Read the model definition and answer for the solid it produces. Units are mm, in the model's axes. Face numbers are marked on the shaded views. Coordinates: 2 decimals unless noted, no trailing zeros. Write each loop counter-clockwise with the first axis right and the second up, starting at its lowest first coordinate (ties: lowest second). Pieces come first, ordered by that corner, then holes.
(1) Section D-D on y = 5.5 is taken. Write down the section's boundary in (x, z), then the cut area to 3 significant figures.
(2) Section C-C on z = -12.25 is taken. Write down the section's boundary in (x, y), then the cut area to 3 significant figures.
(3) The mould has two halves that part along Z. Classify the marked faces 1, 2, 3 and 4: +Z half, -Z half, draft (parallel to the pull), parting line (faces both ways), or undercut.
(4) Section A-A on z = -21 is taken. Write down the section's boundary in (x, y).
(5) Find the intervals of material crossed by probe 1 along Z at (x, y) = (19.5, -16); probe 2 along Z at (x, y) = (-4.5, -15.5); probe 3 along X at (y, z) = (-28, -14), in increasing order.
(6) Given pin 1 (1 mm diameter, centred on y = 26.5, z = -11.5, fed in from -X); pin 2 (4.5 mm diameter, centred on y = -22, z = -20.5, fed in from -X); pin 3 (3 mm diameter, centred on x = -21.5, z = -19, fed in from +Y), each flat-ended and moving along its own axis, determine where each tip first touches the part or whether it passes through.
(7) Section B-B on x = 10.5 is taken. Write down the section's boundary in (y, z).
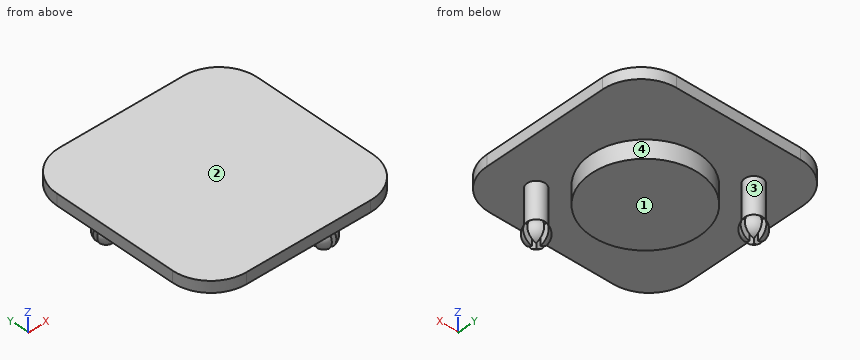
from build123d import *

# Parameters (mm, degrees)
BOX002_W     = 2
BOX002_H     = 12
BOX002_DEPTH = 10
BOX001_W     = 12
BOX001_H     = 2
BOX001_DEPTH = 10
BOX003_W     = 2
BOX003_H     = 12
BOX003_DEPTH = 10
BOX_W        = 12
BOX_H        = 2
BOX_DEPTH    = 10
PAD_DEPTH    = 5
SKETCH001_R  = 24
PAD001_DEPTH = 8
SKETCH002_R  = 4
PAD002_DEPTH = 16


with BuildPart() as cubo002:
    # Box002 → Box002 (new body)
    with BuildSketch(Plane(origin=(-26, 19, -25), x_dir=(1, 0, 0), z_dir=(0, 0, 1))):
        with Locations((1, 6)):
            Rectangle(BOX002_W, BOX002_H)
    extrude(amount=BOX002_DEPTH)


with BuildPart() as fusion:
    # Box001 → Box001 (new body)
    with BuildSketch(Plane(origin=(-31, 24, -25), x_dir=(1, 0, 0), z_dir=(0, 0, 1))):
        with Locations((6, 1)):
            Rectangle(BOX001_W, BOX001_H)
    extrude(amount=BOX001_DEPTH)

    # Fusion: union Cubo002
    add(cubo002.part)


with BuildPart() as cut001:
    # Sphere001 → Sphere001 (revolve)
    with BuildSketch(Plane(origin=(-25, 25, -19), x_dir=(1, 0, 0), z_dir=(0, -1, 0))):
        with BuildLine():
            ThreePointArc((0, -5), (5, 0), (0, 5))
            Line((0, 5), (0, -5))
        make_face()
    revolve(axis=Axis((-25, 25, -19), (0, 0, 1)))

    # Cut001: cut Fusion
    add(fusion.part, mode=Mode.SUBTRACT)


with BuildPart() as cubo003:
    # Box003 → Box003 (new body)
    with BuildSketch(Plane(origin=(24, -31, -25), x_dir=(1, 0, 0), z_dir=(0, 0, 1))):
        with Locations((1, 6)):
            Rectangle(BOX003_W, BOX003_H)
    extrude(amount=BOX003_DEPTH)


with BuildPart() as fusion001:
    # Box → Box (new body)
    with BuildSketch(Plane(origin=(19, -26, -25), x_dir=(1, 0, 0), z_dir=(0, 0, 1))):
        with Locations((6, 1)):
            Rectangle(BOX_W, BOX_H)
    extrude(amount=BOX_DEPTH)

    # Fusion001: union Cubo003
    add(cubo003.part)


with BuildPart() as cut:
    # Sphere → Sphere (revolve)
    with BuildSketch(Plane(origin=(25, -25, -19), x_dir=(1, 0, 0), z_dir=(0, -1, 0))):
        with BuildLine():
            ThreePointArc((0, -5), (5, 0), (0, 5))
            Line((0, 5), (0, -5))
        make_face()
    revolve(axis=Axis((25, -25, -19), (0, 0, 1)))

    # Cut: cut Fusion001
    add(fusion001.part, mode=Mode.SUBTRACT)


with BuildPart() as fusion002:
    # Sketch → Pad (new body)
    with BuildSketch(Plane.XY):
        with BuildLine():
            Line((-27.5, 44.5), (27.5, 44.5))
            ThreePointArc((44.5, 27.5), (39.520815, 39.520815), (27.5, 44.5))
            Line((44.5, 27.5), (44.5, -27.5))
            ThreePointArc((27.5, -44.5), (39.520815, -39.520815), (44.5, -27.5))
            Line((27.5, -44.5), (-27.5, -44.5))
            ThreePointArc((-44.5, -27.5), (-39.520815, -39.520815), (-27.5, -44.5))
            Line((-44.5, -27.5), (-44.5, 27.5))
            ThreePointArc((-27.5, 44.5), (-39.520815, 39.520815), (-44.5, 27.5))
        make_face()
    extrude(amount=PAD_DEPTH)

    # Sketch001 (on Face9 of Pad) → Pad001 (join)
    with BuildSketch(Plane(origin=(0, 0, 0), x_dir=(1, 0, 0), z_dir=(0, 0, -1))):
        with Locations((0.149781, -0.32649)):
            Circle(SKETCH001_R)
    extrude(amount=PAD001_DEPTH)

    # Sketch002 (on Face4 of Pad001) → Pad002 (join)
    with BuildSketch(Plane(origin=(0, 0, 0), x_dir=(1, 0, 0), z_dir=(0, 0, -1))):
        with Locations((25, 25)):
            Circle(SKETCH002_R)
        with Locations((-25, -25)):
            Circle(SKETCH002_R)
    extrude(amount=PAD002_DEPTH)

    # Fusion002: union Cut001, Cut
    add(cut001.part)
    add(cut.part)


solid = fusion002.part
Response:
1. outline: (-44.5, 0) - (-23.29, 0) - (-23.29, -8) - (23.59, -8) - (23.59, 0) - (44.5, 0) - (44.5, 5) - (-44.5, 5) - close
1. area: 820 mm2
2. outline: circle Ø8 at (-25, 25); circle Ø8 at (25, -25)
2. area: 101 mm2
3. face 1: -Z half
3. face 2: +Z half
3. face 3: undercut
3. face 4: draft
4. outline: (-29.47, 24) arc R4.58 ccw to (-26, 20.53) - (-26, 24) - close; (-29.47, 26) - (-26, 26) - (-26, 29.47) arc R4.58 ccw to start; (-24, 20.53) arc R4.58 ccw to (-20.53, 24) - (-24, 24) - close; (-24, 26) - (-20.53, 26) arc R4.58 ccw to (-24, 29.47) - close; (20.53, -26) arc R4.58 ccw to (24, -29.47) - (24, -26) - close; (20.53, -24) - (24, -24) - (24, -20.53) arc R4.58 ccw to start; (26, -29.47) arc R4.58 ccw to (29.47, -26) - (26, -26) - close; (26, -24) - (29.47, -24) arc R4.58 ccw to (26, -20.53) - close
5. probe 1: z = 0 to 5
5. probe 2: z = -8 to 5
5. probe 3: x = 22.35 to 27.65
6. pin 1: stops at x = -28.87
6. pin 2: stops at x = 20.12
6. pin 3: stops at y = 29.58
7. outline: (-44.5, 0) - (-21.33, 0) - (-21.33, -8) - (21.98, -8) - (21.98, 0) - (44.5, 0) - (44.5, 5) - (-44.5, 5) - close
